Verification items for the finished model (mm, model axes). Give positions to 0.01 mm unless a question says otherwise; leave off trailing zeros. Loops run counter-clockwise (first coordinate to the right, second up) from the corner with the lowest first, then second, coordinate; pieces in that order, holes last. Notation, with made-up numbers: (55.25, 2.5) - (98.25, 2.5) arc R18 cw to (98.25, 11.5) - close; hole circle Ø8 at (19, 49.25). An arc over 180 degrees is marked (long way). Use one line per item in the form item = value.
```python
from build123d import *

# Parameters (mm, degrees)
BOSS_EXTRUDE1_START = 33.02
BOSS_EXTRUDE1_DEPTH = 5.08
SKETCH4_R           = 25.4
CUT_EXTRUDE1_DEPTH  = 50.8
CUT_EXTRUDE5_START  = 5.08
SKETCH1_R           = 143.404424797
CUT_EXTRUDE5_DEPTH  = 38.1
CHAMFER1_SIZE2      = 5.08
CHAMFER1_SIZE       = 10.894095156
SKETCH6_W           = 33.782
SKETCH6_H           = 14.432407555
CUT_EXTRUDE7_DEPTH  = 25.4
SKETCH7_R           = 3.175
CUT_EXTRUDE8_DEPTH  = 5.08
SKETCH8_R           = 3.175
CUT_EXTRUDE9_DEPTH  = 5.08


with BuildPart() as part:
    # Sketch2 → Boss-Extrude1 (new body)
    with BuildSketch(Plane(origin=(0, 0, 0), x_dir=(1, 0, 0), z_dir=(0, 1, 0)).offset(BOSS_EXTRUDE1_START)):
        Polygon((-203.2, 381), (-44.423028516, 381), (-44.423028516, 423.747508854), (44.020558762, 423.747508854), (44.020558762, 381), (381, 381), (381, 0), (-203.2, 0), align=None)
    extrude(amount=BOSS_EXTRUDE1_DEPTH)

    # Sketch4 → Cut-Extrude1 (cut)
    with BuildSketch(Plane.XZ.offset(-33.02)):
        with Locations(Location((0, -381, 0), (0, 0, 270))):
            Circle(SKETCH4_R)
    extrude(amount=-CUT_EXTRUDE1_DEPTH, mode=Mode.SUBTRACT)

    # Sketch1 → Cut-Extrude5 (cut)
    with BuildSketch(Plane(origin=(0, 0, 0), x_dir=(1, 0, 0), z_dir=(0, 1, 0)).offset(CUT_EXTRUDE5_START)):
        with Locations((-59.795575203, 143.404424797)):
            Circle(SKETCH1_R)
    extrude(amount=CUT_EXTRUDE5_DEPTH, mode=Mode.SUBTRACT)


with BuildPart() as cut_extrude5_kept_piece:
    # of the separate pieces the step leaves, the one the design keeps (cut_extrude5_pieces_kept)
    add(part.part.solids().sort_by_distance((-203.2, 33.02, -381))[0])

    # Chamfer1
    chamfer1_edges = [cut_extrude5_kept_piece.edges().sort_by_distance(p)[0] for p in [
        (41.606666023, 38.1, -244.806666023),
    ]]
    chamfer1_side = [cut_extrude5_kept_piece.faces().sort_by_distance(p)[0] for p in [
        (41.678508072, 38.1, -244.878508072),
    ]]
    chamfer(chamfer1_edges, length=CHAMFER1_SIZE - 0.0001, length2=CHAMFER1_SIZE2 - 0.0001, reference=chamfer1_side[0])  # a hair under: the kernel refuses the full size

    # Sketch6 → Cut-Extrude7 (cut)
    with BuildSketch(Plane.ZY.offset(203.2)):
        with Locations((-160.295424797, 40.236203778)):
            Rectangle(SKETCH6_W, SKETCH6_H)
    extrude(amount=-CUT_EXTRUDE7_DEPTH, mode=Mode.SUBTRACT)

    # Sketch7 → Cut-Extrude8 (cut)
    with BuildSketch(Plane(origin=(0, 38.1, 0), x_dir=(1, 0, 0), z_dir=(0, 1, 0))):
        with Locations(Location((368.3, 152.4, 0), (0, 0, 270))):
            Circle(SKETCH7_R)
        with Locations(Location((374.65, 279.4, 0), (0, 0, 270))):
            Circle(SKETCH7_R)
        with Locations(Location((332.74, 177.8, 0), (0, 0, 270))):
            Circle(SKETCH7_R)
        with Locations(Location((279.4, 101.6, 0), (0, 0, 270))):
            Circle(SKETCH7_R)
        with Locations(Location((101.6, 6.35, 0), (0, 0, 270))):
            Circle(SKETCH7_R)
        with Locations(Location((203.2, 48.26, 0), (0, 0, 270))):
            Circle(SKETCH7_R)
        with Locations(Location((228.6, 12.7, 0), (0, 0, 270))):
            Circle(SKETCH7_R)
        with Locations(Location((368.3, 12.7, 0), (0, 0, 270))):
            Circle(SKETCH7_R)
    extrude(amount=-CUT_EXTRUDE8_DEPTH, mode=Mode.SUBTRACT)

    # Sketch8 → Cut-Extrude9 (cut)
    with BuildSketch(Plane(origin=(0, 38.1, 0), x_dir=(1, 0, 0), z_dir=(0, 1, 0))):
        with Locations(Location((-190.5, 368.3, 0), (0, 0, 270))):
            Circle(SKETCH8_R)
        with Locations(Location((-116.84, 368.3, 0), (0, 0, 270))):
            Circle(SKETCH8_R)
        with Locations(Location((-83.82, 302.26, 0), (0, 0, 270))):
            Circle(SKETCH8_R)
        with Locations(Location((-142.24, 281.94, 0), (0, 0, 270))):
            Circle(SKETCH8_R)
        with Locations(Location((-190.5, 304.8, 0), (0, 0, 270))):
            Circle(SKETCH8_R)
        with Locations(Location((-190.5, 233.68, 0), (0, 0, 270))):
            Circle(SKETCH8_R)
    extrude(amount=-CUT_EXTRUDE9_DEPTH, mode=Mode.SUBTRACT)


solid = cut_extrude5_kept_piece.part
```
1. Scan lines: probe 1 along Z at (x, y) = (203.2, 35.2) (3 decimals); probe 2 along Z at (x, y) = (368.3, 36.6) (3 decimals); probe 3 along X at (y, z) = (35.3, -304.8) (3 decimals). Record each from-to range of solid material in increasing order.
Result set:
probe_1 = -381 to -51.435, -45.085 to 0
probe_2 = -381 to -155.575, -149.225 to -15.875, -9.525 to 0
probe_3 = -203.2 to -193.675, -187.325 to -85.725, -81.915 to 381
2. Depth check by flat-ended pin: pin 1 Ø7.5 at (x, z) = (-190.5, -233.68) entering from -Y; pin 2 Ø2.5 at (y, z) = (35.5, -410.5) entering from -X; pin 3 Ø2 at (x, y) = (-201, 34) entering from +Z; pin 4 Ø2 at (x, y) = (272, 36) entering from -Z. Enter the tip coordinate at first touch or a pass-through.
Result set:
pin_1 = 33.02
pin_2 = -44.42
pin_3 = -177.19
pin_4 = -381
3. Section check B-B, the plane x = 244. Record the cut outline in (y, z), then the cut area to 3 significant figures.
Result set:
outline = (33.02, -381) - (38.1, -381) - (38.1, 0) - (33.02, 0) - close
area = 1,940 mm²
4. Section check A-A, the plane y = 35.95. State how many separate pieces and enclosed holes the cut face has, then the cut area to 3 significant figures.
Result set:
separate_pieces = 1
enclosed_holes = 15
area = 151,000 mm²
5. Draft check along Z on faces 1 (the cylindrical face through (7.629, 35.524, -405.227)), 2 (the flat face through (158, 33.02, -215)), 3 (the conical face through (50.19, 33.267, -236.249)). Enter one of: released by +Z, released by -Z, zero draft, split by the parting line, or undercut.
Result set:
face_1 = undercut
face_2 = zero draft
face_3 = undercut
